from build123d import *

# Parameters (mm, degrees)
F1_DEPTH = 40


with BuildPart() as f1:
    # F0 (on Top) → F1 (new body)
    with BuildSketch(Plane.XY):
        Polygon((22.5, 17.604167), (0, 17.604167), (0, 22.416667), (0, 23.104167), (-3.5, 23.104167), (-25.5, 23.104167), (-29, 23.104167), (-29, 19.604167), (-29, -8.020833), (-29, -16.395833), (-29, -19.895833), (-25.5, -19.895833), (-3.5, -19.895833), (0, -19.895833), (0, -14.395833), (22.5, -14.395833), align=None)
        Polygon((-3.5, 17.604167), (-3.5, -14.395833), (-3.5, -16.395833), (-25.5, -16.395833), (-25.5, -8.020833), (-25.5, 11.229167), (-25.5, 19.604167), (-3.5, 19.604167), align=None, mode=Mode.SUBTRACT)
        Polygon((19, -10.895833), (0, -10.895833), (0, -10.883333), (0, -8.770833), (0, 14.104167), (19, 14.104167), align=None, mode=Mode.SUBTRACT)
    extrude(amount=F1_DEPTH)


solid = f1.part
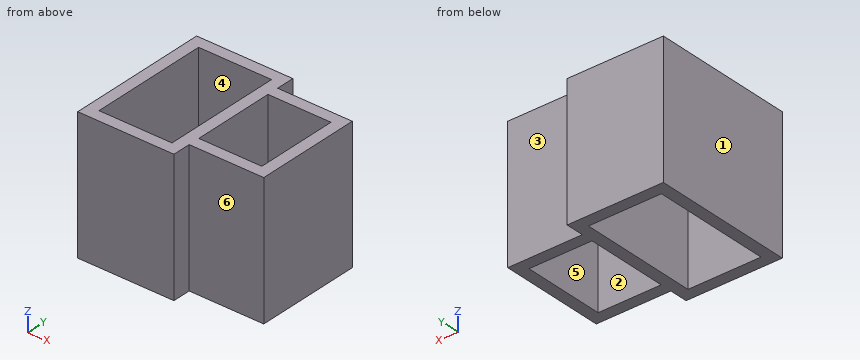
Work out the finished part from the listing and answer in its coordinate system (mm). Face numbers are marked on the shaded views. A direction names the side the tool comes from. Give positions to 0.01 mm unless a question says otherwise; leave off trailing zeros. Order: outer loops, then holes, each group sorted by start corner. A loop starts at its lowest first (then second) coordinate and runs counter-clockwise, first axis right, second up. Notation, with made-up numbers: (-16.5, 53) -> (35.5, 53) arc R9 cw to (35.5, 69) -> close; hole circle Ø11 at (-0.5, -5). An arc over 180 degrees is marked (long way). One line per item, written item: value.
Item 1: Find section D-D, the plane y = 15. Give the vertices of the cut face in (x, z), plus the area to 3 significant figures.
Answer sheet:
outline: (-29, 0) -> (-25.5, 0) -> (-25.5, 40) -> (-29, 40) -> close; (-3.5, 0) -> (22.5, 0) -> (22.5, 40) -> (-3.5, 40) -> close
area: 1,180 mm²
Item 2: A tool of negligible diameter and unlimited length cuts with its end or side. For the marked faces 1 and 2, from which of +Z, -Z, +X, -X, +Y, -Y can it reach the whole face along a straight path? Write none if from no direction.
Answer sheet:
face 1: +Z, -Z, -X, +Y, -Y
face 2: +Z, -Z
Item 3: Flat-ended cylindrical pins translate along their axes: P1, Ø11, axis at x = 14, z = 20.5, coming from the -Y side; P2, Ø5, axis at x = 16, y = 16, coming from the -Z side; P3, Ø11, axis at x = 15.5, z = 27.5, coming from the +Y side; P4, Ø1.5, axis at x = -5.5, y = 17.5, coming from the -Z side. Find the tip coordinate at first contact, or state that the pin passes through.
Answer sheet:
P1: y = -14.4
P2: z = 0
P3: y = 17.6
P4: through
Item 4: Find section C-C, the plane y = -8.5. Give the vertices of the cut face in (x, z).
Answer sheet:
outline: (-29, 0) -> (-25.5, 0) -> (-25.5, 40) -> (-29, 40) -> close; (-3.5, 0) -> (0, 0) -> (0, 40) -> (-3.5, 40) -> close; (19, 0) -> (22.5, 0) -> (22.5, 40) -> (19, 40) -> close
Item 5: Find section B-B, the plane z = 30.5. Give the vertices of the cut face in (x, y), plus the area to 3 significant figures.
Answer sheet:
outline: (-29, -19.9) -> (0, -19.9) -> (0, -14.4) -> (22.5, -14.4) -> (22.5, 17.6) -> (0, 17.6) -> (0, 23.1) -> (-29, 23.1) -> close; hole (-25.5, -16.4) -> (-3.5, -16.4) -> (-3.5, 19.6) -> (-25.5, 19.6) -> close; hole (0, -10.9) -> (19, -10.9) -> (19, 14.1) -> (0, 14.1) -> close
area: 700 mm²
Item 6: Straight lines are drawn through the part: probe 1 along X at (y, z) = (1.5, 38); probe 2 along Y at (x, z) = (13, 6.5); probe 3 along Y at (x, z) = (-15.5, 5.5). For each, find the intervals that lie inside material, in ascending order.
Answer sheet:
probe 1: -29 to -25.5, -3.5 to 0, 19 to 22.5
probe 2: -14.4 to -10.9, 14.1 to 17.6
probe 3: -19.9 to -16.4, 19.6 to 23.1
Item 7: Find section A-A, the plane x = -10.5. Give the vertices of the cut face in (y, z).
Answer sheet:
outline: (-19.9, 0) -> (-16.4, 0) -> (-16.4, 40) -> (-19.9, 40) -> close; (19.6, 0) -> (23.1, 0) -> (23.1, 40) -> (19.6, 40) -> close
Item 8: Determine the mould class of the marked faces 3, 4, 5 and 6 for opening direction Y: released by +Y, released by -Y, zero draft, split by the parting line, or undercut.
Answer sheet:
face 3: released by +Y
face 4: undercut
face 5: undercut
face 6: released by -Y
